Autodesk Inventor part; units mm, degrees
ref_plane "YZ Plane" through (0, 0, 0) normal (1, 0, 0) x (0, 1, 0)
ref_plane "XZ Plane" through (0, 0, 0) normal (0, 1, 0) x (-1, 0, 0)
ref_plane "XY Plane" through (0, 0, 0) normal (0, 0, 1) x (1, 0, 0)
sketch "Sketch1" plane through (0, 0, 0) normal (1, 0, 0) x (0, 1, 0)
  line L0 (0, 0) -> (0, 10)
  line L1 (0, 10) -> (0, 20)
  line L2 (0, 20) -> (0, 30)
  line L3 (0, 30) -> (0, 40)
  line L4 (0, 40) -> (-70, 40)
  line L5 (-70, 40) -> (-70, 0)
  line L6 (-70, 0) -> (0, 0)
  line L7 (0, 0) -> (0, 40)
  line L8 (0, 40) -> (-3, 40)
  line L9 (-3, 40) -> (-3, 30)
  line L10 (-3, 30) -> (-3, 20)
  line L11 (-3, 20) -> (-3, 10)
  line L12 (-3, 10) -> (-3, 0)
  line L13 (-3, 30) -> (0, 30)
  line L14 (-3, 20) -> (0, 20)
  line L15 (-3, 10) -> (0, 10)
  dimension "d0" = 10
  dimension "d1" = 10
  dimension "d2" = 10
  dimension "d3" = 10
  dimension "d4" = 70
  dimension "d5" = 40
  dimension "d6" = 3
  dimension "d7" = 10
  dimension "d8" = 10
  dimension "d9" = 10
  dimension "d10" = 10
extrude "Extrusion1" add sketch "Sketch1" against normal blind 3 contours L6 L12 L15 L0 | L6 L5 L4 L9 L10 L11 L12 | L14 L10 L13 L2
mirror "Mirror1" about plane through (0, -70, 0) normal (0, -1, 0) of "Extrusion1"
properties part number "voorruit"
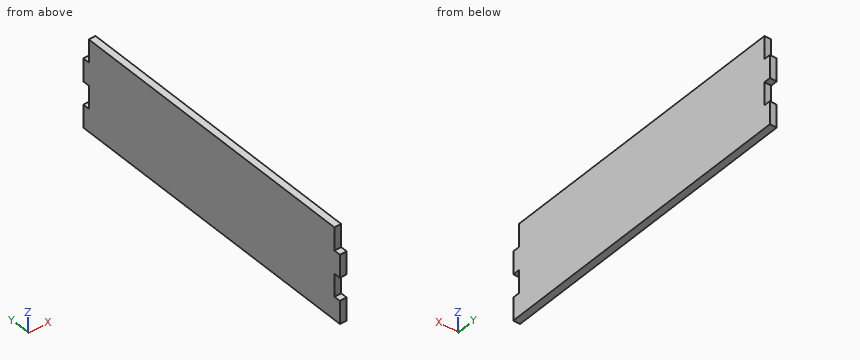
Here's how the part is built. I have some questions about the finished solid (model axes, mm). Give positions to 0.01 mm unless a question says otherwise; leave off trailing zeros. Write each loop counter-clockwise with the first axis right and the second up, starting at its lowest first coordinate (ties: lowest second). Pieces come first, ordered by that corner, then holes. Notation, with made-up numbers: M 4.5,-8 L 50.5,-8 A10 ccw 50.5,-1 Z; hole C -38.75,-21.75 d1. An arc over 180 degrees is marked long. Put each result on its own line as item: value. Start each with the question number.
Item 1: If we section it at B-B, the plane z = 36: Write out the boundary of the cut face in (x, y).
Item 2: I need wall thicknesses on L1, parallel to Y at x = -1.55, z = 34. Which ranges of the line are inside material? Lowest first, please. Write a range as from..to.
Item 3: Will these pins go through, and if not, where does the flat tip stop? pin 1 (1.5 mm diameter, centred on x = -1.5, y = -138, fed in from +Z); pin 2 (1.5 mm diameter, centred on x = -1, z = 13, fed in from +Y); pin 3 (5 mm diameter, centred on y = -36.5, z = 16.5, fed in from +X).
Item 4: If we section it at A-A, the plane x = -2.1: Write out the boundary of the cut face in (y, z), then the cut area to 3 significant figures.
Values:
1. outline: M -3,-137 L 0,-137 L 0,-3 L -3,-3 Z
2. L1: -137..-3
3. pin 1: z = 30
3. pin 2: y = -3
3. pin 3: x = 0
4. outline: M -140,0 L 0,0 L 0,10 L -3,10 L -3,20 L 0,20 L 0,30 L -3,30 L -3,40 L -137,40 L -137,30 L -140,30 L -140,20 L -137,20 L -137,10 L -140,10 Z
4. area: 5,480 mm²
